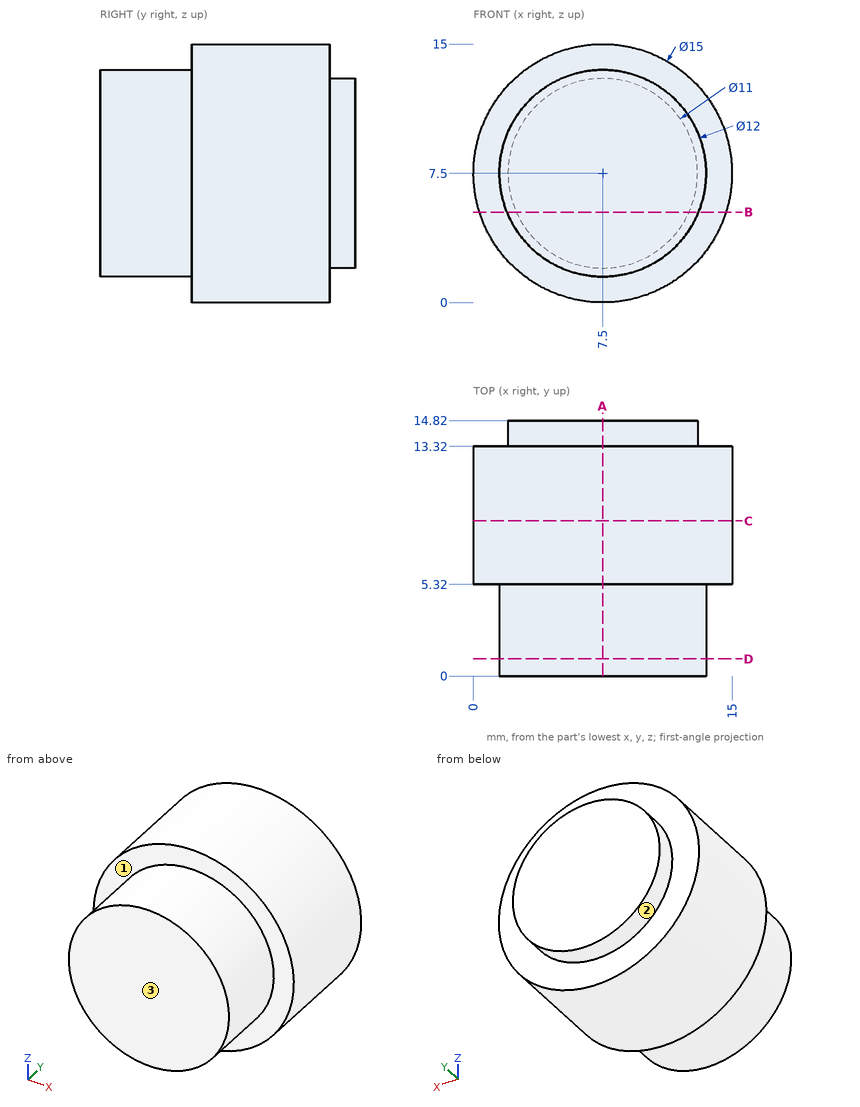
Verification items for this drawing (mm, ordinates from the low corner). A direction names the side the tool comes from. Coordinates: 2 decimals unless noted, no trailing zeros. Order: outer loops, then holes, each group sorted by start corner. A loop starts at its lowest first (then second) coordinate and runs counter-clockwise, first axis right, second up. Notation, with made-up numbers: (56, 32.5) -> (103, 32.5) arc R30 cw to (103, 59.5) -> close; hole circle Ø11 at (8.5, 36). An arc over 180 degrees is marked (long way). Put each result on its own line as item: value. Start each with the question number.
1. Cross-section at D-D, the plane y = 1. Record the boundary of the cut face in (x, z), then the cut area to 3 significant figures.
2. Cross-section at C-C, the plane y = 9. Record the boundary of the cut face in (x, z).
3. Material ranges on L1, parallel to Y at x = 2.5, z = 3; L2, parallel to Z at x = 3, y = 12; L3, parallel to Y at x = 6.25, z = 13, recorded low to high. Write a range as [from, to].
4. Cross-section at B-B, the plane z = 5.25. Record the boundary of the cut face in (x, y).
5. Go/stop test with flat-tipped pins: pin 1 Ø1 at (x, z) = (11.5, 9) entering from -Y; pin 2 Ø1.5 at (x, y) = (6, 13) entering from +Z; pin 3 Ø3 at (y, z) = (6.5, 2) entering from +X; pin 4 Ø2 at (x, y) = (5, 11.5) entering from +Z. Record where each tip stops, or that it passes through.
6. Access from +Z, -Z, +X, -X, +Y, -Y to the whole of each face (thin tool, end or side, straight path). Record for the marked faces 1, 2 and 3.
7. Cross-section at A-A, the plane x = 7.5. Record the boundary of the cut face in (y, z).
Computed:
1. outline: circle Ø12 at (7.5, 7.5)
1. area: 113 mm2
2. outline: circle Ø15 at (7.5, 7.5)
3. L1: [5.32, 13.32]
3. L2: [1.5, 13.5]
3. L3: [0, 13.32]
4. outline: (0.35, 5.32) -> (1.94, 5.32) -> (1.94, 0) -> (13.06, 0) -> (13.06, 5.32) -> (14.65, 5.32) -> (14.65, 13.32) -> (12.52, 13.32) -> (12.52, 14.82) -> (2.48, 14.82) -> (2.48, 13.32) -> (0.35, 13.32) -> close
5. pin 1: y = 0
5. pin 2: z = 14.96
5. pin 3: x = 13.84
5. pin 4: z = 14.85
6. face 1: -Y
6. face 2: +Y
6. face 3: +Z, -Z, +X, -X, -Y
7. outline: (0, 1.5) -> (5.32, 1.5) -> (5.32, 0) -> (13.32, 0) -> (13.32, 2) -> (14.82, 2) -> (14.82, 13) -> (13.32, 13) -> (13.32, 15) -> (5.32, 15) -> (5.32, 13.5) -> (0, 13.5) -> close
